The listing builds one solid part. Answer for the finished solid, in the listing's coordinates (mm). A direction names the side the tool comes from. Round coordinates to 2 decimals unless told otherwise and drop trailing zeros. Loops run counter-clockwise (first coordinate to the right, second up) from the corner with the lowest first, then second, coordinate; pieces in that order, holes last. Notation, with made-up numbers: (-1.5, -36.75) -> (16.5, -36.75) arc R19 cw to (16.5, -10.75) -> close; hole circle Ø1 at (26.25, -39). An arc over 180 degrees is marked (long way). Write each question's results on one line, items separated by ' | '. Start each with the question number.
(1) Straight lines are drawn through the part: probe 1 along Z at (x, y) = (-25, -4.25); probe 2 along X at (y, z) = (-10, -5); probe 3 along X at (y, z) = (-6, 4.75). For each, find the intervals that lie inside material, in ascending order.
(2) Determine the mould class of faces 1 (the face through (-27, -6, -9)), 2 (the face through (29, -6.8, 5)), 3 (the face through (8.96, -9.32, 2.82)) for opening direction Y: released by +Y, released by -Y, zero draft, split by the parting line, or undercut.
(3) The part is cut by section D-D (x = -25). Determine the outline of the cut face in (y, z), plus the area to 3 significant figures.
(4) The part is cut by section B-B (z = 4.75). Determine the outline of the cut face in (x, y), plus the area to 3 significant figures.
(5) The part is cut by section A-A (x = 12). Determine the outline of the cut face in (y, z).
(6) The part is cut by section C-C (y = -6). Count the separate pieces of the cut face and the enclosed holes in it, plus the area to 3 significant figures.
(7) For faces 4 (the face through (-26.652, -3.448, 10.246)), 5 (the face through (14, -3, 8)), 6 (the face through (21.5, -5.9, -7)), 7 (the face through (-25, -4, -5)), determine the directions among +Z, -Z, +X, -X, +Y, -Y from which every point of the face is accessible in a straight line to the end or side of a thin tool.
(8) Flat-ended cylindrical pins translate along their axes: pin 1 (6 mm diameter, centred on x = -12, y = -6, fed in from +Z); pin 2 (4.5 mm diameter, centred on x = -11, y = -7, fed in from -Z); pin 3 (10.5 mm diameter, centred on x = -25, z = 5, fed in from +Y); pin 4 (1 mm diameter, centred on x = -8, y = -5, fed in from -Z). Find the tip coordinate at first contact, or state that the pin passes through.
Autodesk Inventor part; units mm, degrees
ref_plane "YZ Plane" through (0, 0, 0) normal (1, 0, 0) x (0, 1, 0)
ref_plane "XZ Plane" through (0, 0, 0) normal (0, 1, 0) x (-1, 0, 0)
ref_plane "XY Plane" through (0, 0, 0) normal (0, 0, 1) x (1, 0, 0)
sketch "Sketch1" plane through (0, 0, 0) normal (0, 1, 0) x (-1, 0, 0)
  line L0 (40.6019, 0) -> (-40.6019, 0) construction
  line L1 (0, 14.7427) -> (0, -14.7427) construction
  line L2 (25, 5) -> (-25, 5) construction
  line L3 (-25, 5) -> (-25, -5) construction
  line L4 (-25, -5) -> (25, -5) construction
  line L5 (25, -5) -> (25, 5) construction
  line L6 (34, 13) -> (-34, 13)
  line L7 (-34, 13) -> (-34, -9)
  line L8 (-34, -9) -> (34, -9)
  line L9 (34, -9) -> (34, 13)
  line L10 (26, -5) -> (24, -5) construction
  line L11 (26, -3) -> (24, -3)
  line L12 (24, -7) -> (26, -7)
  arc A0 (26, -7) -> (26, -3) centre (26, -5) ccw
  arc A1 (24, -3) -> (24, -7) centre (24, -5) ccw
  point P0 (0, 0)
  point P1 (0, 0)
  point P2 (-25, 5)
  dimension "d2" = 50
  dimension "d3" = 10
  dimension "d4" = 68
  dimension "d5" = 22
  dimension "d16" = 8
  dimension "d17" = 1
  dimension "d18" = 4
extrude "Extrusion1" add sketch "Sketch1" against normal blind 12 contours L9 L8 L7 L6 | A0 L12 A1 L11
sketch "Sketch6" plane through (0, -12, 0) normal (0, -1, 0) x (1, 0, 0)
  line L0 (-26, -3) -> (-24, -3)
  arc A0 (-26, -3) -> (-26, -7) centre (-26, -5) ccw
  line L1 (-24, -7) -> (-26, -7)
  arc A1 (-24, -7) -> (-24, -3) centre (-24, -5) ccw
  point P0 (0, 0)
  point P1 (25, -5)
hole "Hole5" at (25, -12, -5) direction (0, 1, 0) diameter 4 depth 8 tip angle 118
extrude "Extrusion4" cut sketch "Sketch6" against normal blind 8
hole "Hole1" at (-25, 0, 5) at (25, 0, 5) direction (0, -1, 0) diameter 6.6 end through all counterbore diameter 11 counterbore depth 6.8
sketch "Sketch3" plane through (0, 0, 0) normal (0, 1, 0) x (1, 0, 0)
  line L0 (19.5, 9) -> (-19.5, 9)
  line L1 (-19.5, 9) -> (-19.5, 3)
  line L2 (-19.5, 3) -> (19.5, 3)
  line L3 (19.5, 3) -> (19.5, 9)
  line L4 (34, 9) -> (-34, 9)
  line L5 (0, 0) -> (0, 9) construction
  dimension "d34" = 39
  dimension "d35" = 6
extrude "Extrusion2" cut sketch "Sketch3" against normal through all
chamfer "Chamfer2" distance 4 angle 45 6 edges at (34, -6, -9) (34, -6, 13) (-34, -6, 13) (-34, -6, -9) (19.5, -6, -9) (-19.5, -6, -9)
fillet "Fillet2" radius 1.5 2 edges at (-19.5, -6, -3) (19.5, -6, -3)
sketch "Sketch7" plane through (18, 0, -3) normal (0, 0, -1) x (-1, 0, 0)
  line L0 (18, 0) -> (18, -12)
  line L1 (-12, -12) -> (48, -12)
  line L2 (30, -6) -> (6, -6)
  point P0 (18, -6)
  dimension "d67" = 24
hole "Hole6" at (-12, -6, -3) at (12, -6, -3) direction (0, 0, 1) diameter 6.5 end through all counterbore diameter 9 counterbore depth 11
chamfer "Chamfer3" distance 0.5 angle 45 2 edges at (12, -10.5, -3) (-12, -10.5, -3)
equation "\"d67\" = shaftSeparation"
equation "\"shaftSeparation\" = 24"
properties part number "FAB-OX002x-PiezoPusherBaseComponent" material "Aluminum 6061"
Checked values:
1) probe 1: z = -9 to -7, -3 to -0.5, 10.5 to 13 | probe 2: x = -34 to -28, -22 to -19.5, 19.5 to 23, 27 to 34 | probe 3: x = -34 to -30.49, -19.51 to -16.5, -7.5 to 7.5, 16.5 to 19.51, 30.49 to 34
2) face 1: zero draft | face 2: released by +Y | face 3: undercut
3) outline: (-12, -9) -> (0, -9) -> (0, -0.5) -> (-6.8, -0.5) -> (-6.8, 1.7) -> (-12, 1.7) -> (-12, -3) -> (-4, -3) -> (-4, -7) -> (-12, -7) -> close; (-12, 8.3) -> (-6.8, 8.3) -> (-6.8, 10.5) -> (0, 10.5) -> (0, 13) -> (-12, 13) -> close | area: 123 mm2
4) outline: (-34, -12) -> (-28.29, -12) -> (-28.29, -6.8) -> (-30.49, -6.8) -> (-30.49, 0) -> (-34, 0) -> close; (-21.71, -12) -> (21.71, -12) -> (21.71, -6.8) -> (19.51, -6.8) -> (19.51, 0) -> (-19.51, 0) -> (-19.51, -6.8) -> (-21.71, -6.8) -> close; (28.29, -12) -> (34, -12) -> (34, 0) -> (30.49, 0) -> (30.49, -6.8) -> (28.29, -6.8) -> close; hole circle Ø9 at (-12, -6); hole circle Ø9 at (12, -6) | area: 471 mm2
5) outline: (-12, -3) -> (-11, -3) -> (-10.5, -2.5) -> (-10.5, 8) -> (-9.25, 8) -> (-9.25, 13) -> (-12, 13) -> close; (-2.75, 8) -> (-1.5, 8) -> (-1.5, -2.5) -> (-1, -3) -> (0, -3) -> (0, 13) -> (-2.75, 13) -> close
6) separate pieces: 3 | enclosed holes: 4 | area: 728 mm2
7) face 4: +Y | face 5: -Z | face 6: -Z, +Y, -Y | face 7: -Y
8) pin 1: passes through | pin 2: stops at z = 8 | pin 3: stops at y = -6.8 | pin 4: stops at z = -2.62
